from build123d import *

# Parameters (mm, degrees)
SKETCH1_W           = 7
SKETCH1_H           = 7
BOSS_EXTRUDE1_DEPTH = 1
SKETCH2_W           = 1.02
SKETCH2_H           = 1.02
BOSS_EXTRUDE2_DEPTH = 5.5
SKETCH4_R           = 3
BOSS_EXTRUDE3_DEPTH = 16
CHAMFER1_SIZE       = 0.6


with BuildPart() as part:
    # Sketch1 → Boss-Extrude1 (new body)
    with BuildSketch(Plane(origin=(0, 0, 0), x_dir=(1, 0, 0), z_dir=(0, 1, 0))):
        Rectangle(SKETCH1_W, SKETCH1_H)
    extrude(amount=BOSS_EXTRUDE1_DEPTH)

    # Sketch2 → Boss-Extrude2 (add)
    with BuildSketch(Plane.XZ):
        with Locations((-2.54, 2.129508614)):
            Rectangle(SKETCH2_W, SKETCH2_H)
        with Locations((-2.54, -2.129508614)):
            Rectangle(SKETCH2_W, SKETCH2_H)
        with Locations((2.54, 2.129508614)):
            Rectangle(SKETCH2_W, SKETCH2_H)
        with Locations((2.54, -2.129508614)):
            Rectangle(SKETCH2_W, SKETCH2_H)
    extrude(amount=BOSS_EXTRUDE2_DEPTH)

    # Sketch4 → Boss-Extrude3 (add)
    with BuildSketch(Plane(origin=(0, 1, 0), x_dir=(1, 0, 0), z_dir=(0, 1, 0))):
        with Locations(Location((0, 0, 0), (0, 0, 270))):
            Circle(SKETCH4_R)
    extrude(amount=BOSS_EXTRUDE3_DEPTH)

    # Chamfer1
    chamfer1_edges = [part.edges().sort_by_distance(p)[0] for p in [
        (0, 17, -3),
    ]]
    chamfer(chamfer1_edges, length=CHAMFER1_SIZE)


solid = part.part
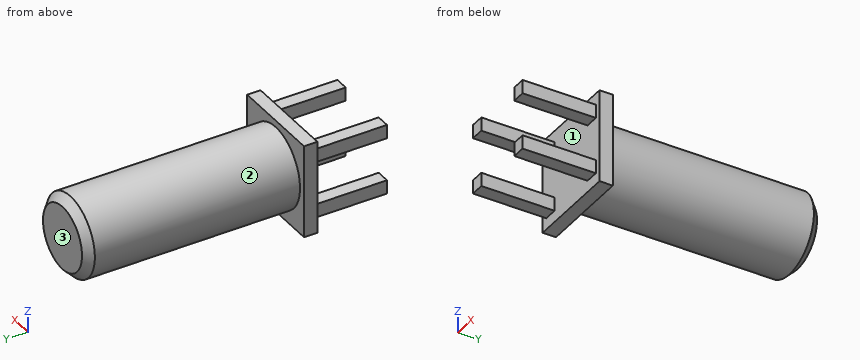
Part model, mm, in its own coordinate system. Face numbers are marked on the shaded views. Give positions to 0.01 mm unless a question says otherwise; leave off trailing zeros. Order: outer loops, then holes, each group sorted by start corner. A loop starts at its lowest first (then second) coordinate and runs counter-clockwise, first axis right, second up. Notation, with made-up numbers: (40.25, -33) - (73.25, -33) arc R22 cw to (73.25, -22) - close; hole circle Ø1 at (45.25, -13). An arc over 180 degrees is marked (long way). One line per question, with ' | ' between items.
1. Pull direction X, two halves, no side cores. Call the marked faces 1, 2 and 3: +X half, -X half, draft (parallel to the pull), parting line (faces both ways), or undercut.
Filled in:
face 1: undercut | face 2: parting line | face 3: draft
2. Band-saw the part on C-C on z = 0. List the corners of the cut face in (x, y), then the cut area to 3 significant figures.
Filled in:
outline: (-3.5, 0) - (3.5, 0) - (3.5, 1) - (3, 1) - (3, 16.4) - (2.4, 17) - (-2.4, 17) - (-3, 16.4) - (-3, 1) - (-3.5, 1) - close | area: 103 mm²
3. Drop flat-ended pins along their axis: P1, Ø3, axis at x = -2.5, z = 0, coming from the -Y side; P2, Ø1.5, axis at y = 2, z = 2.5, coming from the -X side; P3, Ø0.8, axis at y = -1.5, z = -2, coming from the -X side. Give the stop position or say it passes through.
Filled in:
P1: y = 0 | P2: x = -2.44 | P3: x = -3.05
4. Band-saw the part on B-B on x = 0. List the corners of the cut face in (y, z).
Filled in:
outline: (0, -3.5) - (1, -3.5) - (1, -3) - (16.4, -3) - (17, -2.4) - (17, 2.4) - (16.4, 3) - (1, 3) - (1, 3.5) - (0, 3.5) - close
5. Band-saw the part on A-A on y = -3.5. List the corners of the cut face in (x, z), then the cut area to 3 significant figures.
Filled in:
outline: (-3.05, -2.64) - (-2.03, -2.64) - (-2.03, -1.62) - (-3.05, -1.62) - close; (-3.05, 1.62) - (-2.03, 1.62) - (-2.03, 2.64) - (-3.05, 2.64) - close; (2.03, -2.64) - (3.05, -2.64) - (3.05, -1.62) - (2.03, -1.62) - close; (2.03, 1.62) - (3.05, 1.62) - (3.05, 2.64) - (2.03, 2.64) - close | area: 4.16 mm²
6. Band-saw the part on D-D on y = 3.5. List the corners of the cut face in (x, z), then the cut area to 3 significant figures.
Filled in:
outline: circle Ø6 at (0, 0) | area: 28.3 mm²
7. Drill centre lines: probe 1 along X at (y, z) = (-2, -2.25); probe 2 along Z at (x, y) = (-2.5, -4); probe 3 along Y at (x, z) = (1, 1.75). Where is each one in solid material? Low to high.
Filled in:
probe 1: -3.05 to -2.03, 2.03 to 3.05 | probe 2: -2.64 to -1.62, 1.62 to 2.64 | probe 3: 0 to 17
